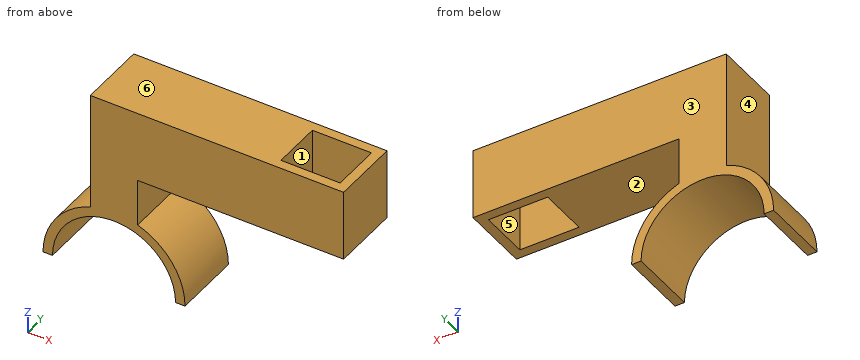
```python
from build123d import *

# Parameters (mm, degrees)
SKETCH1_W           = 16.5
SKETCH1_H           = 14.5
SKETCH1_W_2         = 12.5
SKETCH1_H_2         = 10.5
BOSS_EXTRUDE1_DEPTH = 15
SKETCH2_W           = 15
SKETCH2_H           = 14.5
BOSS_EXTRUDE2_DEPTH = 37
SKETCH3_W           = 10
SKETCH3_H           = 14.5
BOSS_EXTRUDE3_DEPTH = 10
BOSS_EXTRUDE4_DEPTH = 14.5


with BuildPart() as part:
    # Sketch1 → Boss-Extrude1 (new body)
    with BuildSketch(Plane.XY):
        with Locations((6.25, -5.25)):
            Rectangle(SKETCH1_W, SKETCH1_H)
        with Locations((6.25, -5.25)):
            Rectangle(SKETCH1_W_2, SKETCH1_H_2, mode=Mode.SUBTRACT)
    extrude(amount=BOSS_EXTRUDE1_DEPTH)

    # Sketch2 → Boss-Extrude2 (add)
    with BuildSketch(Plane.ZY.offset(2)):
        with Locations((7.5, -5.25)):
            Rectangle(SKETCH2_W, SKETCH2_H)
    extrude(amount=BOSS_EXTRUDE2_DEPTH)

    # Sketch3 → Boss-Extrude3 (add)
    with BuildSketch(Plane(origin=(0, 0, 0), x_dir=(-1, 0, 0), z_dir=(0, 0, -1))):
        with Locations((34, -5.25)):
            Rectangle(SKETCH3_W, SKETCH3_H)
    extrude(amount=BOSS_EXTRUDE3_DEPTH)

    # Sketch4 → Boss-Extrude4 (add)
    with BuildSketch(Plane(origin=(0, 2, 0), x_dir=(1, 0, 0), z_dir=(0, 1, 0))):
        with BuildLine():
            Line((-19, 24.142135624), (-21, 24.142135624))
            ThreePointArc((-21, 24.142135624), (-34, 11.142135624), (-47, 24.142135624))
            Line((-47, 24.142135624), (-49, 24.142135624))
            ThreePointArc((-49, 24.142135624), (-34, 9.142135624), (-19, 24.142135624))
        make_face()
    extrude(amount=-BOSS_EXTRUDE4_DEPTH)


solid = part.part
```
Read the model definition and answer for the solid it produces. Units are mm, in the model's axes. Face numbers are marked on the shaded views. A direction names the side the tool comes from. Coordinates: 2 decimals unless noted, no trailing zeros. Loops run counter-clockwise (first coordinate to the right, second up) from the corner with the lowest first, then second, coordinate; pieces in that order, holes last.
(1) The part is cut by section B-B (z = 11). Determine the outline of the cut face in (x, y).
Solution:
outline: (-39, -12.5) - (14.5, -12.5) - (14.5, 2) - (-39, 2) - close; hole (0, -10.5) - (12.5, -10.5) - (12.5, 0) - (0, 0) - close
(2) A tool of negligible diameter and unlimited length cuts with its end or side. For the marked faces 1, 2 and 3, from which of +Z, -Z, +X, -X, +Y, -Y can it reach the whole face along a straight path? Write none if from no direction.
Solution:
face 1: +Z, -Z
face 2: +X, +Y, -Y
face 3: +Z, -Z, +X, -X, +Y
(3) Consider line 1 along X through (y, z) = (-1.75, 4); line 2 along Z through (x, y) = (-10.5, -6); line 3 along X through (y, z) = (-10.75, 13.5). Determine where each line is inside the solid, lowest interval first.
Solution:
line 1: x = -39 to 0, 12.5 to 14.5
line 2: z = 0 to 15
line 3: x = -39 to 14.5
(4) The part is cut by section A-A (y = -8). Determine the outline of the cut face in (x, z).
Solution:
outline: (-49, -24.14) - (-47, -24.14) arc R13 cw to (-21, -24.14) - (-19, -24.14) arc R15 ccw to (-29, -10) - (-29, 0) - (0, 0) - (0, 15) - (-39, 15) - (-39, -10) arc R15 ccw to start; (12.5, 0) - (14.5, 0) - (14.5, 15) - (12.5, 15) - close
(5) Flat-ended cylindrical pins translate along their axes: pin 1 Ø1 at (y, z) = (0.5, -11) entering from +X; pin 2 Ø4.5 at (y, z) = (-6.5, 0) entering from -X. Find the tip coordinate at first contact, or state that the pin passes through.
Solution:
pin 1: stops at x = -25.93
pin 2: stops at x = -39
(6) The part is cut by section D-D (x = -15.5). Determine the outline of the cut face in (y, z), and give its area (4 significant figures).
Solution:
outline: (-12.5, 0) - (2, 0) - (2, 15) - (-12.5, 15) - close
area: 217.5 mm2
(7) The part is cut by section C-C (z = -17). Determine the outline of the cut face in (x, y), and give its area (3 significant figures).
Solution:
outline: (-47.19, -12.5) - (-44.86, -12.5) - (-44.86, 2) - (-47.19, 2) - close; (-23.14, -12.5) - (-20.81, -12.5) - (-20.81, 2) - (-23.14, 2) - close
area: 67.5 mm2
(8) The mould has two halves that part along X. Classify the marked faces 4, 5 and 6: released by +X, released by -X, zero draft, split by the parting line, or undercut.
Solution:
face 4: released by -X
face 5: undercut
face 6: zero draft
